The listing builds one solid part. Answer for the finished solid, in the listing's coordinates (mm). Coordinates: 2 decimals unless noted, no trailing zeros. Write each loop counter-clockwise with the first axis right and the second up, starting at its lowest first coordinate (ties: lowest second). Pieces come first, ordered by that corner, then holes.
(1) The part is cut by section D-D on y = -2. Determine the outline of the cut face in (x, z), plus the area to 3 significant figures.
(2) Straight lines are drawn through the part: line 1 (Z direction, x = 0, y = 4.75); line 2 (X direction, y = -13, z = 38); line 3 (Y direction, x = 55, z = -7.5). For each, find the intervals that lie inside material, in ascending order.
(3) The part is cut by section A-A on z = 30. Determine the outline of the cut face in (x, y).
(4) The part is cut by section C-C on x = 28.5. Determine the outline of the cut face in (y, z).
(5) Given P1, Ø0.9, axis at x = 60.5, y = 24, coming from the -Z side; P2, Ø21.5, axis at x = 0, z = 0.04, coming from the -Y side; P3, Ø3, axis at y = -40.5, z = 30, coming from the -X side, each flat-ended and moving along its own axis, determine where each tip first touches the part or whether it passes through.
(6) The part is cut by section B-B on x = 3. Determine the outline of the cut face in (y, z).
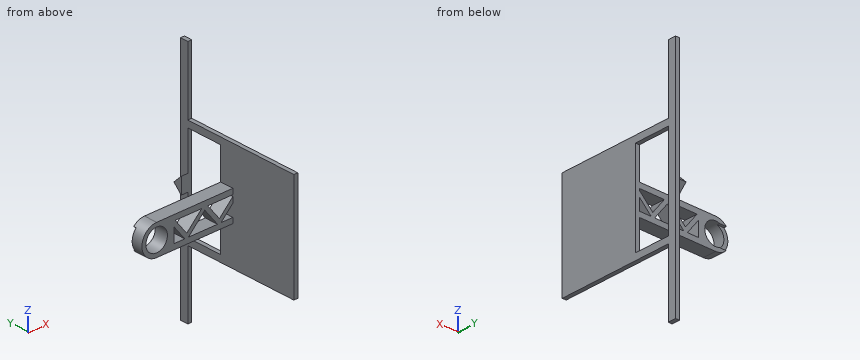
Autodesk Inventor part; units mm, degrees
ref_plane "YZ Plane" through (0, 0, 0) normal (1, 0, 0) x (0, 1, 0)
ref_plane "XZ Plane" through (0, 0, 0) normal (0, 1, 0) x (-1, 0, 0)
ref_plane "XY Plane" through (0, 0, 0) normal (0, 0, 1) x (1, 0, 0)
sketch "Sketch1" plane through (0, 0, 0) normal (0, 1, 0) x (-1, 0, 0)
  line L0 (-122.594, 12.25) -> (-122.594, -12.2908)
  line L1 (-61.296, -11.2083) -> (-61.296, 11.2917)
  line L2 (0, 0) -> (-13.1, 0)
  line L3 (-61.296, 0) -> (-63.296, 0)
  circle A0 centre (0, 0.0417) radius 8.25
  arc A1 (0, -11.2083) -> (0, 11.2917) centre (0, 0.0417) ccw
  line L4 (0, -11.2083) -> (-61.296, -11.2083)
  line L5 (0, 11.2917) -> (-61.296, 11.2917)
  dimension "d24" = 61.296
  dimension "d28" = 16.5
  dimension "d30" = 3
extrude "Extrusion1" add sketch "Sketch1" along normal blind 10
sketch "Sketch3" plane through (0, 10, 0) normal (0, 1, 0) x (1, 0, 0)
  line L0 (8.1183, -12.2504) -> (8.1163, 12.2496)
  line L1 (13.1167, 7.25) -> (13.1179, -7.25)
  line L2 (39.1319, -7.25) -> (47.9899, 4.2277)
  line L3 (36.5087, -5.7388) -> (46.5328, 7.25)
  line L4 (49.2102, 7.25) -> (62.1991, -5.7388)
  line L5 (13.1179, -7.25) -> (61.3127, -7.25)
  line L6 (61.296, -11.2917) -> (61.296, 11.2083)
  line L7 (13.1167, 7.25) -> (61.3127, 7.25)
  line L8 (61.3127, -7.25) -> (61.3127, 7.25)
  line L9 (47.9899, 4.2277) -> (59.4676, -7.25)
  line L10 (61.296, -9.1202) -> (61.4899, -9.3141)
  line L11 (49.2102, 7.25) -> (61.296, -4.8775)
  line L12 (13.1179, -7.25) -> (21.1056, -7.25)
  line L13 (21.1056, 7.25) -> (13.1179, 7.25)
  line L14 (13.1179, 7.25) -> (13.1179, -7.25)
  line L15 (24.1056, -7.25) -> (33.7772, -7.25)
  line L16 (21.1057, 5.5674) -> (21.1056, 5.5673)
  line L17 (23.5198, 7.25) -> (23.5198, -7.25)
  line L18 (36.5087, -5.7388) -> (35.3424, -7.25)
  line L19 (11.5087, -5.7388) -> (10.3424, -7.25)
  line L20 (11.5087, -5.7388) -> (21.5328, 7.25)
  line L21 (14.1319, -7.25) -> (22.9899, 4.2277)
  line L22 (22.9899, 4.2277) -> (34.4676, -7.25)
  line L23 (24.2102, 7.25) -> (36.296, -4.8775)
  line L24 (24.2102, 7.25) -> (37.1991, -5.7388)
  line L25 (36.3127, -7.25) -> (36.3127, 7.25)
  line L26 (36.296, -9.1202) -> (36.4899, -9.3141)
  point P0 (0, 0)
  point P1 (0, 0)
  point P2 (61.297, -12.25)
  point P3 (61.295, 12.2704)
  point P4 (62.1991, -5.7388)
  point P5 (61.2954, 7.25)
  point P6 (61.296, -4.8358)
  point P7 (61.296, -7.25)
  point P8 (61.296, 7.25)
  point P9 (13.1179, -1.906)
  point P10 (36.8094, -5.3492)
  point P11 (13.1179, -3.6537)
  point P12 (21.5328, 7.25)
  dimension "d9" = 5
  dimension "d53" = 25
extrude "Extrusion2" cut sketch "Sketch3" against normal blind 10 contours L7 L20 L1 | L21 L22 L17 L5 | L7 L25 L24 | L22 L5 L17 | L7 L3 L24 L25 | L7 L6 L4 | L2 L9 L5
sketch "Sketch7" plane through (0, 10, 0) normal (0, 1, 0) x (1, 0, 0)
  circle A0 centre (0, 0) radius 62.296
  dimension "d20" = 124.592
sketch "Sketch8" plane through (61.296, 0, 12.25) normal (1, 0, 0) x (0, 0, -1)
  line L0 (-27.75, 0) -> (52.25, 0)
  line L1 (52.25, 0) -> (52.25, 10)
  line L2 (52.25, 10) -> (-27.75, 10)
  line L3 (-27.75, 10) -> (-27.75, 0)
  line L4 (-27.75, 0) -> (52.25, 10) construction
  line L5 (52.25, 0) -> (-27.75, 10) construction
  line L6 (52.25, 10) -> (-27.75, 10)
  line L7 (-27.75, 10) -> (-27.75, -50)
  line L8 (-27.75, -50) -> (52.25, -50)
  line L9 (52.25, -50) -> (52.25, 10)
  line L10 (52.25, 10) -> (47.25, 10)
  line L11 (47.25, 10) -> (47.25, 37)
  line L12 (-27.75, 10) -> (52.25, 10)
  line L13 (-27.75, 37) -> (-27.75, 10)
  line L14 (-27.75, 10) -> (-22.75, 10)
  line L15 (-22.75, 10) -> (-22.75, 37)
  line L16 (-22.75, 37) -> (47.25, 37)
  line L17 (52.25, 43) -> (-27.75, 43)
  line L18 (-30.75, 10.375) -> (-30.75, 10)
  line L19 (-77.7917, 37) -> (-77.7917, 43)
  line L20 (-77.7917, 43) -> (102.2083, 43)
  line L21 (102.2083, 43) -> (102.2083, 37)
  line L22 (102.2083, 37) -> (-77.7917, 43) construction
  line L23 (-77.7917, 37) -> (102.2083, 43) construction
  line L24 (-27.75, 37) -> (-77.7917, 37)
  line L25 (52.25, 10) -> (52.25, 37)
  line L26 (52.25, 37) -> (52.25, 10)
  line L27 (102.2083, 37) -> (52.25, 37)
  line L28 (47.25, 37) -> (-22.75, 37)
  line L29 (23.4583, 10) -> (0.9583, 10)
  line L30 (12.2083, 10) -> (12.2083, 37)
  point P0 (12.25, 0)
  point P1 (47.25, 10)
  point P2 (-57.7845, 37.6669)
  point P3 (47.25, 10)
  point P4 (12.2083, 40)
  dimension "d21" = 80
  dimension "d34" = 60
  dimension "d41" = 5
  dimension "d44" = 180
  dimension "d58" = 0
extrude "Extrusion4" add sketch "Sketch8" against normal blind 3 contours L3 L2 L1 L0 | L0 L9 L8 L7 | L13 L24 L19 L20 L17 L21 L27 L25 L2 L11 L16 L15
sketch "Sketch11" plane through (0, 10, 0) normal (0, 1, 0) x (1, 0, 0)
  circle A0 centre (0, -0.0417) radius 8.25
  line L0 (-3.0682, -7.7) -> (-14.6805, -7.7)
  line L1 (-14.6805, -7.7) -> (-14.6805, 7.7)
  line L2 (-14.6805, 7.7) -> (-3.0682, 7.7)
  line L3 (-3.0682, 7.7) -> (-3.0682, 7.6165)
  line L4 (-3.0682, -7.7) -> (0, -7.7)
  line L5 (0, -7.7) -> (0, -0.0417)
  line L6 (0, -0.0417) -> (0, 7.7)
  line L7 (0, 7.7) -> (-3.0682, 7.7)
  point P0 (0, 0)
  point P1 (-4.1158, 7.1083)
  point P2 (-2.8509, 7.7)
  dimension "d39" = 15.4
  dimension "d40" = 7.7
extrude "Extrusion6" cut sketch "Sketch11" against normal blind 2 contours L3 L7 A0 | A0 L0 L1 L2 L3 | L4 L5 L6 L7 A0 picked at (0.9906, 5.1042)
sketch "Sketch12" plane through (58.296, 0, 12.25) normal (-1, 0, 0) x (0, 0, 1)
  point P0 (-12.25, 0)
sketch "Sketch14" plane through (58.296, 0, 12.25) normal (-1, 0, 0) x (0, 0, 1)
  line L0 (-102.2083, 43) -> (77.7917, 43)
  line L1 (22.75, 37) -> (-47.25, 37)
  line L2 (-12.2083, 43) -> (-16.882, 38.3262)
  line L3 (-12.2083, 43) -> (-5.5985, 43) construction
  line L4 (-16.882, 38.3262) -> (-18.25, 37)
  line L5 (-12.2083, 43) -> (-7.0615, 37.8533)
  line L6 (-12.2083, 43) -> (-4.9297, 43) construction
  line L7 (-7.0615, 37.8533) -> (-6.2083, 37)
  line L8 (-6.2083, 37) -> (-18.25, 37)
  point P0 (-12.25, 0)
  dimension "d45" = 135
  dimension "d46" = 45
extrude "Extrusion7" add sketch "Sketch14" along normal blind 5
properties part number "Tower"
Model answer:
1. outline: (58.3, -40) - (61.3, -40) - (61.3, 40) - (58.3, 40) - close
1. area: 240 mm2
2. line 1: z = -11.21 to -8.21, 8.29 to 11.29
2. line 2: x = 58.3 to 61.3
2. line 3: y = 0 to 10
3. outline: (58.3, -50) - (61.3, -50) - (61.3, 10) - (58.3, 10) - close; (58.3, 37) - (61.3, 37) - (61.3, 43) - (58.3, 43) - close
4. outline: (0, -11.21) - (10, -11.21) - (10, -7.25) - (0, -7.25) - close; (0, -2.96) - (10, -2.96) - (10, 1.28) - (0, 1.28) - close; (0, 7.25) - (10, 7.25) - (10, 11.29) - (0, 11.29) - close
5. P1: stops at z = -40
5. P2: stops at y = 0
5. P3: stops at x = 58.3
6. outline: (0, -11.21) - (10, -11.21) - (10, -7.64) - (0, -7.64) - close; (0, 7.73) - (10, 7.73) - (10, 11.29) - (0, 11.29) - close
